```python
from build123d import *

# Parameters (mm, degrees)
SKETCH1_W             = 8
SKETCH1_H             = 8
BOSS_EXTRUDE1_DEPTH   = 4
FILLET1_R             = 0.4
SKETCH3_R             = 1.6
CUT_EXTRUDE1_DEPTH    = 5
SKETCH4_W             = 5.4
SKETCH4_H             = 5.4
SKETCH4_R             = 1.6
CUT_EXTRUDE2_DEPTH    = 2.6
CHAMFER1_SIZE         = 0.2
CHAMFER1_SIZE2        = 0.346410162
CHAMFER1_PART_2_SIZE  = 0.2
CHAMFER1_PART_2_SIZE2 = 0.346410162
CHAMFER1_PART_3_SIZE  = 0.2
CHAMFER1_PART_3_SIZE2 = 0.346410162
CHAMFER1_PART_4_SIZE  = 0.2
CHAMFER1_PART_4_SIZE2 = 0.346410162
CHAMFER1_PART_5_SIZE  = 0.2
CHAMFER1_PART_5_SIZE2 = 0.346410162
CHAMFER1_PART_6_SIZE  = 0.2
CHAMFER1_PART_6_SIZE2 = 0.346410162


with BuildPart() as part:
    # Sketch1 → Boss-Extrude1 (new body)
    with BuildSketch(Plane.XY):
        Rectangle(SKETCH1_W, SKETCH1_H)
    extrude(amount=BOSS_EXTRUDE1_DEPTH)

    # Fillet1
    fillet1_edges = [part.edges().sort_by_distance(p)[0] for p in [
        (-4, 4, 2),
        (4, 4, 2),
        (4, -4, 2),
        (-4, -4, 2),
    ]]
    fillet(fillet1_edges, radius=FILLET1_R)

    # Sketch3 → Cut-Extrude1 (cut, through all)
    with BuildSketch(Plane(origin=(0, 0, 0), x_dir=(-1, 0, 0), z_dir=(0, 0, -1))):
        Circle(SKETCH3_R)
    extrude(amount=-CUT_EXTRUDE1_DEPTH, mode=Mode.SUBTRACT)

    # Sketch4 → Cut-Extrude2 (cut)
    with BuildSketch(Plane.XY.offset(4)):
        Rectangle(SKETCH4_W, SKETCH4_H)
        with Locations(Location((0, 0, 0), (0, 0, 180))):  # turned: the seam where the file's is
            Circle(SKETCH4_R, mode=Mode.SUBTRACT)
    extrude(amount=-CUT_EXTRUDE2_DEPTH, mode=Mode.SUBTRACT)

    # Chamfer1
    chamfer1_edges = [part.edges().sort_by_distance(p)[0] for p in [
        (0, -4, 0),
        (-4, 0, 0),
        (0, 4, 0),
        (4, 0, 0),
        (-3.882842712, 3.882842712, 0),
        (3.882842712, 3.882842712, 0),
        (3.882842712, -3.882842712, 0),
        (-3.882842712, -3.882842712, 0),
        (1.6, 0, 0),
    ]]
    chamfer1_side = [part.faces().sort_by_distance(p)[0] for p in [
        (0, 3.886862915, 0),
    ]]
    chamfer(chamfer1_edges, length=CHAMFER1_SIZE, length2=CHAMFER1_SIZE2, reference=chamfer1_side[0])

    # Chamfer1 part 2
    chamfer1_part_2_edges = [part.edges().sort_by_distance(p)[0] for p in [
        (0, -4, 4),
        (-4, 0, 4),
        (4, 0, 4),
        (0, 4, 4),
        (-3.882842712, 3.882842712, 4),
        (3.882842712, 3.882842712, 4),
        (3.882842712, -3.882842712, 4),
        (-3.882842712, -3.882842712, 4),
    ]]
    chamfer1_part_2_side = [part.faces().sort_by_distance(p)[0] for p in [
        (0, 3.886862915, 4),
    ]]
    chamfer(chamfer1_part_2_edges, length=CHAMFER1_PART_2_SIZE, length2=CHAMFER1_PART_2_SIZE2, reference=chamfer1_part_2_side[0])

    # Chamfer1 part 3
    chamfer1_part_3_edges = [part.edges().sort_by_distance(p)[0] for p in [
        (-2.7, 0, 4),
    ]]
    chamfer1_part_3_side = [part.faces().sort_by_distance(p)[0] for p in [
        (-2.7, 0, 2.7),
    ]]
    chamfer(chamfer1_part_3_edges, length=CHAMFER1_PART_3_SIZE, length2=CHAMFER1_PART_3_SIZE2, reference=chamfer1_part_3_side[0])

    # Chamfer1 part 4
    chamfer1_part_4_edges = [part.edges().sort_by_distance(p)[0] for p in [
        (0, -2.7, 4),
    ]]
    chamfer1_part_4_side = [part.faces().sort_by_distance(p)[0] for p in [
        (0, -2.7, 2.7),
    ]]
    chamfer(chamfer1_part_4_edges, length=CHAMFER1_PART_4_SIZE, length2=CHAMFER1_PART_4_SIZE2, reference=chamfer1_part_4_side[0])

    # Chamfer1 part 5
    chamfer1_part_5_edges = [part.edges().sort_by_distance(p)[0] for p in [
        (2.7, 0, 4),
    ]]
    chamfer1_part_5_side = [part.faces().sort_by_distance(p)[0] for p in [
        (2.7, 0, 2.7),
    ]]
    chamfer(chamfer1_part_5_edges, length=CHAMFER1_PART_5_SIZE, length2=CHAMFER1_PART_5_SIZE2, reference=chamfer1_part_5_side[0])

    # Chamfer1 part 6
    chamfer1_part_6_edges = [part.edges().sort_by_distance(p)[0] for p in [
        (0, 2.7, 4),
    ]]
    chamfer1_part_6_side = [part.faces().sort_by_distance(p)[0] for p in [
        (0, 2.7, 2.7),
    ]]
    chamfer(chamfer1_part_6_edges, length=CHAMFER1_PART_6_SIZE, length2=CHAMFER1_PART_6_SIZE2, reference=chamfer1_part_6_side[0])


solid = part.part
```
Can you work these out from the model? Positions are in its coordinate system, mm. A direction names the side the tool comes from. Give positions to 0.01 mm unless a question says otherwise; leave off trailing zeros. Loops run counter-clockwise (first coordinate to the right, second up) from the corner with the lowest first, then second, coordinate; pieces in that order, holes last. Notation, with made-up numbers: M 32,76 L 71,76 A23 ccw 71,94 Z; hole C -18,16 d6. An arc over 180 degrees is marked long. Use CSV: the item, a comma, the result in double quotes. Start each with the question number.
1. Imagine slicing it at C-C, the plane z = 1.55. Write out the boundary of the cut face in (x, y), plus the area to 3 significant figures.
2. If I drill on L1, parallel to Y at x = 0.25, z = 3.6; L2, parallel to Y at x = 0, z = 1.05, over which ranges is the centre line in solid material (lowest first)?
3. If we mould it in two halves opening along X, with no side actions, what happens to faces 3 (the face through (1.27, -0.97, 0.87)), 4 (the face through (-4, 0, 2)), 5 (the face through (2, 1, 0))? For each: released by +X, released by -X, zero draft, split by the parting line, or undercut.
4. For P1, Ø2, axis at x = 1, y = 0.5, coming from the +Z side; P2, Ø1.9, axis at x = 0, y = 0, coming from the -Z side, each with a flat end and sliding along its axis, tell me the tip position at first contact or that it passes through.
5. On a 3-axis mill with a long thin cutter (end or side, diameter ignored), from which of +Z, -Z, +X, -X, +Y, -Y can I reach the whole of each face in a straight line? I mean faces 1 (the face through (-1.24, 1.24, 1.4)), 2 (the face through (0, 4, 2)). Say none if no direction works.
6. Imagine slicing it at A-A, the plane x = 0. Write out the boundary of the cut face in (y, z).
7. Imagine slicing it at B-B, the plane y = -2.5. Write out the boundary of the cut face in (x, z).
Response values:
1,outline,"M -4,-3.6 A0.4 ccw -3.6,-4 L 3.6,-4 A0.4 ccw 4,-3.6 L 4,3.6 A0.4 ccw 3.6,4 L -3.6,4 A0.4 ccw -4,3.6 Z; hole M -2.7,-2.7 L 2.7,-2.7 L 2.7,2.7 L -2.7,2.7 Z"
1,area,"34.7 mm^2"
2,L1,"-4 to -2.7, 2.7 to 4"
2,L2,"-4 to -1.6, 1.6 to 4"
3,face 3,"undercut"
3,face 4,"released by -X"
3,face 5,"zero draft"
4,P1,"z = 1.4"
4,P2,"through"
5,face 1,"+Z"
5,face 2,"+Z, -Z, +X, -X, +Y"
6,outline,"M -4,0.35 L -3.8,0 L -1.8,0 L -1.6,0.35 L -1.6,1.4 L -2.7,1.4 L -2.7,3.8 L -3.05,4 L -3.8,4 L -4,3.65 Z; M 1.6,0.35 L 1.8,0 L 3.8,0 L 4,0.35 L 4,3.65 L 3.8,4 L 3.05,4 L 2.7,3.8 L 2.7,1.4 L 1.6,1.4 Z"
7,outline,"M -4,0.35 L -3.8,0 L 3.8,0 L 4,0.35 L 4,3.65 L 3.8,4 L 3.05,4 L 2.7,3.8 L 2.7,1.4 L -2.7,1.4 L -2.7,3.8 L -3.05,4 L -3.8,4 L -4,3.65 Z"
